from build123d import *

# Parameters (mm, degrees)
BOSS_EXTRUDE1_DEPTH = 6.5
SKETCH3_R           = 4.75
BOSS_EXTRUDE2_DEPTH = 25
CHAMFER1_SIZE       = 0.5
CHAMFER2_SIZE       = 0.3


with BuildPart() as part:
    # Sketch1 → Boss-Extrude1 (new body)
    with BuildSketch(Plane(origin=(0, 0, 0), x_dir=(1, 0, 0), z_dir=(0, 1, 0))):
        Polygon((0, 9.237604307), (-8, 4.618802154), (-8, -4.618802154), (0, -9.237604307), (8, -4.618802154), (8, 4.618802154), align=None)
    extrude(amount=-BOSS_EXTRUDE1_DEPTH)

    # Sketch2 → Cut-Revolve1 (revolve, cut)
    with BuildSketch(Plane.XY):
        Polygon((-11, -1.5), (-8, 0), (-8, 1), (-11, 1), align=None)
    cut_revolve1 = revolve(axis=Axis((0, 50, 0), (0, -1, 0)), mode=Mode.SUBTRACT)

    # Sketch3 → Boss-Extrude2 (add)
    with BuildSketch(Plane.XZ.offset(6.5)):
        with Locations(Location((0, 0, 0), (0, 0, 270))):
            Circle(SKETCH3_R)
    extrude(amount=BOSS_EXTRUDE2_DEPTH)

    # Chamfer1
    chamfer1_edges = [part.edges().sort_by_distance(p)[0] for p in [
        (0, -31.5, 4.75),
    ]]
    chamfer(chamfer1_edges, length=CHAMFER1_SIZE)

    # Mirror1: Cut-Revolve1 across plane
    add(cut_revolve1.mirror(Plane(origin=(0, -3.25, 0), x_dir=(0, 0, 1), z_dir=(0, -1, 0))), mode=Mode.SUBTRACT)

    # Chamfer2
    chamfer2_edges = [part.edges().sort_by_distance(p)[0] for p in [
        (0, -6.5, 4.75),
    ]]
    chamfer(chamfer2_edges, length=CHAMFER2_SIZE)


solid = part.part
Build history of the part. All positions in model axes, mm. A direction names the side the tool comes from. Give positions to 0.01 mm unless a question says otherwise; leave off trailing zeros. Order: outer loops, then holes, each group sorted by start corner. A loop starts at its lowest first (then second) coordinate and runs counter-clockwise, first axis right, second up. Notation, with made-up numbers: M 66.5,50 L 112.5,50 A25 ccw 112.5,72 Z; hole C 55.5,23 d3. An arc over 180 degrees is marked long. Put each result on its own line as item: value.
Item 1: Wall check: probe 1 along X at (y, z) = (-21, -0.25); probe 2 along Y at (x, z) = (-2.75, -3.25); probe 3 along Y at (x, z) = (-3.5, 5). Give the ranges that are in metal, low to high.
Results are:
probe 1: -4.74 to 4.74
probe 2: -31.49 to 0
probe 3: -6.5 to 0
Item 2: Which spindle directions (+Z, -Z, +X, -X, +Y, -Y) get a long thin tool onto all of the face, cutting with end or side? Do faces 5 (the face through (-7.174, -6.352, 4.165)), 6 (the face through (-0.1, -6.5, 5.2)). Say none if no direction does.
Results are:
face 5: +Z, -X, -Y
face 6: -Y
Item 3: Pull direction Z, two halves, no side cores. Call faces 1 (the face through (-4.056, -3.205, 6.896)), 2 (the face through (-2.89, -18.73, 3.77)), 3 (the face through (0, 0, 0)), 4 (the face through (7.174, -6.352, -4.165)): +Z half, -Z half, draft (parallel to the pull), parting line (faces both ways), or undercut.
Results are:
face 1: +Z half
face 2: parting line
face 3: draft
face 4: -Z half
Item 4: Cut at A-A on y = -11.5. Write the cut outline in (x, z).
Results are:
outline: C 0,0 d9.5
Item 5: Drop flat-ended pins along their axis: pin 1 Ø2 at (x, y) = (4.5, -17) entering from +Z; pin 2 Ø5 at (x, z) = (4, 7) entering from -Y; pin 3 Ø5 at (x, y) = (4.5, -19) entering from -Z. Give the stop position or say it passes through.
Results are:
pin 1: z = 3.21
pin 2: y = -6.5
pin 3: z = -4.31
